from build123d import *

# Parameters (mm, degrees)
SKETCH_1_R          = 6
EXTRUDE_1_DEPTH     = 6
CUT_EXTRUDE_1_DEPTH = 10


with BuildPart() as part:
    # 草图1 → 凸台-拉伸1 (new body)
    with BuildSketch(Plane.XY):
        with BuildLine():
            Line((0, 9), (105, 9))
            ThreePointArc((105, 9), (114, 0), (105, -9))
            Line((105, -9), (0, -9))
            ThreePointArc((0, -9), (-9, 0), (0, 9))
        make_face()
        Circle(SKETCH_1_R, mode=Mode.SUBTRACT)
        with Locations((105, 0)):
            Circle(SKETCH_1_R, mode=Mode.SUBTRACT)
    extrude(amount=EXTRUDE_1_DEPTH)

    # 草图2 → 切除-拉伸1 (cut)
    with BuildSketch(Plane.XY.offset(6)):
        with BuildLine():
            Line((15, 3.5), (90, 3.5))
            ThreePointArc((90, 3.5), (93.5, 0), (90, -3.5))
            Line((90, -3.5), (15, -3.5))
            ThreePointArc((15, -3.5), (11.5, 0), (15, 3.5))
        make_face()
    extrude(amount=-CUT_EXTRUDE_1_DEPTH, mode=Mode.SUBTRACT)


solid = part.part
Design review of the part built by this model. Coordinates are the model's own, in mm. A direction names the side the tool comes from. Round coordinates to 2 decimals unless told otherwise and drop trailing zeros. Loops run counter-clockwise (first coordinate to the right, second up) from the corner with the lowest first, then second, coordinate; pieces in that order, holes last. Notation, with made-up numbers: M 68.25,1 L 117.25,1 A22 ccw 117.25,26 Z; hole C 40.25,-18.5 d9. An arc over 180 degrees is marked long. Answer as a JSON object with one key per item and string values.
Item 1: The part is to be moulded in two halves that separate along Y. For faces 3 (the cylindrical face through (99, 0, 3)), 4 (the flat face through (53, -4, 6)), 5 (the cylindrical face through (114, 0, 3)), say which applies: pulls with the +Y half, pulls with the -Y half, needs draft (parallel to the pull), parting line crosses it, or undercut.
Answer sheet:
{"face 3": "undercut", "face 4": "needs draft", "face 5": "parting line crosses it"}
Item 2: We need section B-B on y = 0. Give the boundary of the cut face in (x, z).
Answer sheet:
{"outline": "M -9,0 L -6,0 L -6,6 L -9,6 Z; M 6,0 L 11.5,0 L 11.5,6 L 6,6 Z; M 93.5,0 L 99,0 L 99,6 L 93.5,6 Z; M 111,0 L 114,0 L 114,6 L 111,6 Z"}
Item 3: We need section A-A on x = 59.5. Give the boundary of the cut face in (y, z).
Answer sheet:
{"outline": "M -9,0 L -3.5,0 L -3.5,6 L -9,6 Z; M 3.5,0 L 9,0 L 9,6 L 3.5,6 Z"}
Item 4: Machinability: for faces 1 (the cylindrical face through (-9, 0, 3)), 2 (the cylindrical face through (93.5, 0.1, 3)), which of the approach directions +Z, -Z, +X, -X, +Y, -Y give a long, thin tool a straight path to every point of the face, cutting with its end or side? Answer none if there is none.
Answer sheet:
{"face 1": "+Z, -Z, -X", "face 2": "+Z, -Z"}
Item 5: We need section D-D on y = 5. Give the boundary of the cut face in (x, z), and give its area (3 significant figures).
Answer sheet:
{"outline": "M -7.48,0 L -3.32,0 L -3.32,6 L -7.48,6 Z; M 3.32,0 L 101.68,0 L 101.68,6 L 3.32,6 Z; M 108.32,0 L 112.48,0 L 112.48,6 L 108.32,6 Z", "area": "640 mm^2"}
Item 6: We need section C-C on z = 4. Give the boundary of the cut face in (x, y), and give its area (3 significant figures).
Answer sheet:
{"outline": "M 0,-9 L 105,-9 A9 ccw 105,9 L 0,9 A9 ccw Z; hole C 0,0 d12; hole M 15,-3.5 L 90,-3.5 A3.5 ccw 90,3.5 L 15,3.5 A3.5 ccw Z; hole C 105,0 d12", "area": "1,350 mm^2"}
Item 7: Clearance check with flat-ended pins moving along their axes: P1, Ø3, axis at y = -5, z = 2.5, coming from the +X side; P2, Ø1, axis at y = 2.5, z = 1.5, coming from the +X side. State where each tip first meets the part, or that it passes through.
Answer sheet:
{"P1": "stops at x = 113.29", "P2": "stops at x = 113.77"}
Item 8: Wall thickness on L1, parallel to Y at x = 51, z = 3.3; L2, parallel to Y at x = 105, z = 3.35; L3, parallel to X at y = 5.5, z = 1.9: over which ranges is each line inside the solid? List them lowest first. Write a range as from..to.
Answer sheet:
{"L1": "y = -9..-3.5, 3.5..9", "L2": "y = -9..-6, 6..9", "L3": "x = -7.12..-2.4, 2.4..102.6, 107.4..112.12"}
